The model under review builds one solid part; all positions refer to its coordinate system, in mm. A direction names the side the tool comes from. Give positions to 0.01 mm unless a question says otherwise; leave off trailing zeros. Loops run counter-clockwise (first coordinate to the right, second up) from the corner with the lowest first, then second, coordinate; pieces in that order, holes last. Notation, with made-up numbers: (-0.5, -38) - (56.5, -38) arc R17 cw to (56.5, -24) - close; hole circle Ø11 at (66.25, 78). An arc over 180 degrees is marked (long way). Return JSON: item names as keys, results as strings. Group by question number.
```python
from build123d import *

# Parameters (mm, degrees)
F1_DEPTH = 17
F2_T     = 2
F3_R     = 6.5480863362
F3_R_2   = 6.2456314412
F3_R_3   = 6.7864098422
F4_DEPTH = 30


with BuildPart() as f1:
    # F0 (on Top) → F1 (new body)
    with BuildSketch(Plane.XY):
        Polygon((-23.5533174127, 36.1492224038), (-33.3842672408, 26.9327051938), (-32.5650200248, -21.8124184757), (-23.1436938047, -30.8241229504), (0, -30.8241229504), (8.397269994, -21.6076094657), (8.397269994, -6.8611833267), (-5.9395320714, -6.8611833267), (-5.9395320714, -13.824773021), (-8.8068926707, -16.2825100124), (-15.7704818994, -16.2825100124), (-18.6378415674, -13.4151503444), (-18.6378415674, 19.3546824157), (-16.5897272527, 21.4027967304), (-7.5780232437, 21.4027967304), (-5.1202862523, 18.9450588077), (-5.1202862523, 14.6440193057), (8.6020808667, 14.6440193057), (8.6020808667, 26.9327051938), (0, 36.1492224038), align=None)
    extrude(amount=F1_DEPTH)

    # F2
    f2_openings = [f1.faces().sort_by_distance(p)[0] for p in [
        (-27.928164, 30.964293, 17),
    ]]
    offset(amount=F2_T, openings=f2_openings, kind=Kind.INTERSECTION)

    # F3 (on face) → F4 (cut)
    with BuildSketch(Plane(origin=(0, 0, -2), x_dir=(1, 0, 0), z_dir=(0, 0, -1))):
        with Locations((-3.3998074941, -27.5282841176)):
            Circle(F3_R)
        with Locations((-26.31444484, -4.339881707)):
            Circle(F3_R_2)
        with Locations((-3.4494721331, 22.0593828708)):
            Circle(F3_R_3)
    extrude(amount=-F4_DEPTH, mode=Mode.SUBTRACT)


solid = f1.part
```
1) Draft analysis for pull direction X (two halves, no side actions). For faces 1 (the face through (-29.323, -27.681, 7.367)), 2 (the face through (4.14, -26.28, 8.38)), 3 (the face through (-18, 0, 17)), state which applies: +X half, -X half, draft (parallel to the pull), parting line (faces both ways), or undercut.
2) We need section D-D, the plane y = 31.5. Write out the cut boundary in (x, z).
3) To check wall thickness, follow line 1 (Y direction, x = -5, z = 8); line 2 (Y direction, x = -10, z = 6.5); line 3 (X direction, y = -9.5, z = 10.5). State the ranges of each line that lie inside material, in increasing order.
4) We need section C-C, the plane x = -3. Write out the cut boundary in (y, z).
5) We need section B-B, the plane y = -11. Write out the cut boundary in (x, z).
6) For pin 1 Ø10 at (x, z) = (-28, 4.5) entering from -Y; pin 2 Ø5 at (x, y) = (-22.5, 14) entering from +Z; pin 3 Ø4.5 at (y, z) = (16, 10.5) entering from -X; pin 4 Ø12 at (x, y) = (-3.45, -22.06) entering from +Z, all flat-tipped, find the tip position at first contact; note any pin that passes through.
7) Tool access review of faces 4 (the face through (1, -4.861, 7)), 5 (the face through (10.397, -14, 7)), 6 (the face through (-12, 36.149, 8)), 7 (the face through (-7.94, -9, 7)): name each direction out of +Z, -Z, +X, -X, +Y, -Y from which nothing blocks a thin tool from reaching the whole face with its end or side.
8) We need section A-A, the plane x = -30.5. Write out the cut boundary in (y, z).
Findings:
{
 "1": {"face 1": "-X half", "face 2": "undercut", "face 3": "draft"},
 "2": {"outline": "(-31.44, -2) - (-8.61, -2) - (-8.61, 0) - (-28.51, 0) - (-28.51, 17) - (-31.44, 17) - close; (1.81, -2) - (7.08, -2) - (7.08, 17) - (4.34, 17) - (4.34, 0) - (1.81, 0) - close"},
 "3": {"line 1": "y = -32.82 to -30.82, -6.86 to -4.86, 12.64 to 14.64, 36.15 to 38.15", "line 2": "y = -32.82 to -30.82, -16.28 to -14.28, 19.4 to 21.4, 36.15 to 38.15", "line 3": "x = -34.77 to -32.77, -18.64 to -16.64, -7.94 to -5.94, 8.4 to 10.4"},
 "4": {"outline": "(-32.82, -2) - (-28.83, -2) - (-28.83, 0) - (-30.82, 0) - (-30.82, 17) - (-32.82, 17) - close; (-15.29, -2) - (-4.86, -2) - (-4.86, 17) - (-6.86, 17) - (-6.86, 0) - (-15.29, 0) - close; (12.64, -2) - (20.99, -2) - (20.99, 0) - (14.64, 0) - (14.64, 17) - (12.64, 17) - close; (34.06, -2) - (38.15, -2) - (38.15, 17) - (36.15, 17) - (36.15, 0) - (34.06, 0) - close"},
 "5": {"outline": "(-34.75, -2) - (-16.64, -2) - (-16.64, 17) - (-18.64, 17) - (-18.64, 0) - (-32.75, 0) - (-32.75, 17) - (-34.75, 17) - close; (-7.94, -2) - (10.4, -2) - (10.4, 17) - (8.4, 17) - (8.4, 0) - (-5.94, 0) - (-5.94, 17) - (-7.94, 17) - close"},
 "6": {"pin 1": "stops at y = -32.82", "pin 2": "stops at z = 0", "pin 3": "stops at x = -35.24", "pin 4": "passes through"},
 "7": {"face 4": "+Z, -Z, +X", "face 5": "+Z, -Z, +X, -Y", "face 6": "+Z", "face 7": "+Z, -Z"},
 "8": {"outline": "(-26.56, -2) - (-0.3, -2) - (-0.3, 0) - (-23.79, 0) - (-23.79, 17) - (-26.56, 17) - close; (8.98, -2) - (32.38, -2) - (32.38, 17) - (29.64, 17) - (29.64, 0) - (8.98, 0) - close"}
}
